from build123d import *

# Parameters (mm, degrees)
F0_R            = 60.325
F0_R_2          = 12.5
F1_DEPTH        = 10
F2_DEPTH        = 12.5
F3_DEPTH        = 12.5
F3_COPIES_COUNT = 26
F4_R            = 12.5
F5_DEPTH        = 22.501
F5_COPIES_COUNT = 5


# Not quite as in the source:
# - a pattern or mirror of a feature is missing from the dataset's text; its kind, count and spacing are read off the source's solid


with BuildPart() as f1:
    # F0 (on Front) → F1 (new body, symmetric)
    with BuildSketch(Plane.XZ):
        with BuildLine():
            ThreePointArc((-5.9714194874, 63.2186060373), (-42.7379507145, -46.9650675367), (63.5, 0))
            ThreePointArc((63.5, 0), (47.6226622583, 42.0039526644), (7.9304869469, 63.0028362598))
            ThreePointArc((7.9304869469, 63.0028362598), (0.9854569889, 63.4923528822), (-5.9714194874, 63.2186060373))
        make_face()
        Circle(F0_R, mode=Mode.SUBTRACT)
        Circle(F0_R)
        Circle(F0_R_2, mode=Mode.SUBTRACT)
    extrude(amount=F1_DEPTH, both=True)

    # F0 (on Front) → F2 (join, symmetric)
    with BuildSketch(Plane.XZ):
        with BuildLine():
            ThreePointArc((-5.9714194874, 63.2186060373), (-42.7379507145, -46.9650675367), (63.5, 0))
            ThreePointArc((63.5, 0), (47.6226622583, 42.0039526644), (7.9304869469, 63.0028362598))
            ThreePointArc((7.9304869469, 63.0028362598), (0.9854569889, 63.4923528822), (-5.9714194874, 63.2186060373))
        make_face()
        Circle(F0_R, mode=Mode.SUBTRACT)
    extrude(amount=F2_DEPTH, both=True)

    # F0 (on Front) → F3 (join, symmetric)
    with BuildSketch(Plane.XZ):
        with BuildLine():
            ThreePointArc((-5.9714194874, 63.2186060373), (0.9854569889, 63.4923528822), (7.9304869469, 63.0028362598))
            Line((7.9304869469, 63.0028362598), (2.54, 78.4059613943))
            Line((2.54, 78.4059613943), (0, 78.4059613943))
            Line((0, 78.4059613943), (-5.9714194874, 63.2186060373))
        make_face()
    f3 = extrude(amount=F3_DEPTH, both=True)

    # F3_copies: F3 ×26 about axis
    f3_copies_axis = Axis((0, 0, 0), (0, 1, 0))
    for i in range(1, F3_COPIES_COUNT):
        add(f3.rotate(f3_copies_axis, i * 360 / F3_COPIES_COUNT))

    # F4 (on face) → F5 (cut, through all)
    with BuildSketch(Plane.XZ.offset(10)):
        with Locations((-30, 0)):
            Circle(F4_R)
    f5 = extrude(amount=-F5_DEPTH, mode=Mode.SUBTRACT)

    # F5_copies: F5 ×5 about axis
    f5_copies_axis = Axis((0, 0, 0), (0, 1, 0))
    for i in range(1, F5_COPIES_COUNT):
        add(f5.rotate(f5_copies_axis, i * 360 / F5_COPIES_COUNT), mode=Mode.SUBTRACT)


solid = f1.part
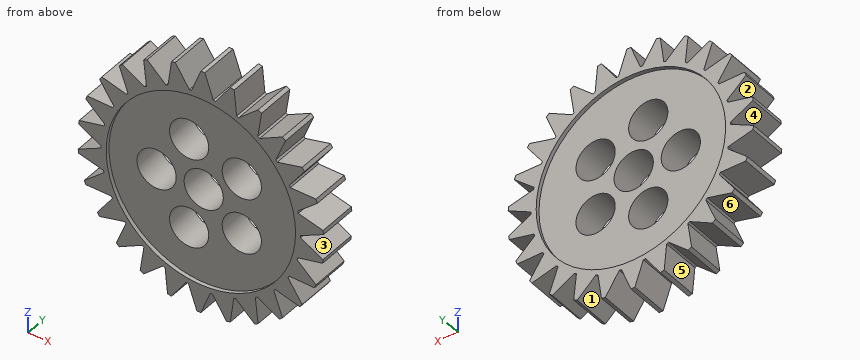
Can you work these out from the model? Positions are in its coordinate system, mm. Face numbers are marked on the shaded views. A direction names the side the tool comes from. Coordinates: 2 decimals unless noted, no trailing zeros. Write each loop counter-clockwise with the first axis right and the second up, starting at its lowest first coordinate (ties: lowest second). Pieces come first, ordered by that corner, then holes. Notation, with made-up numbers: (17, -7.5) -> (51, -7.5) arc R4 cw to (51, -3.5) -> close; hole circle Ø2 at (84.25, 53). An arc over 180 degrees is marked (long way). Write item = value, one per line.
(1) Imagine slicing it at B-B (y = 0). State how many separate pieces and enclosed holes the cut face has, and give its area (3 significant figures).
Verdict:
separate_pieces = 1
enclosed_holes = 6
area = 12,900 mm^2
(2) For pin 1 (8 mm diameter, centred on x = 56.5, y = -0.5, fed in from +Z); pin 2 (12 mm diameter, centred on x = 22.5, y = -5, fed in from -Z); pin 3 (1.5 mm diameter, centred on y = -8, z = 3.5, fed in from -X), each with a flat end and sliding along its axis, tell me the tip position at first contact or that it passes through.
Verdict:
pin_1 = 58.24
pin_2 = -76.69
pin_3 = -68.21
(3) If I drill on probe 1 along X at (y, z) = (0.75, 1); probe 2 along Z at (x, y) = (-58, -4.5); probe 3 along Z at (x, y) = (-57, 4.25), over which ranges is the centre line in solid material (lowest first)?
Verdict:
probe_1 = -63.49 to -42.46, -17.54 to -12.46, 12.46 to 66.1
probe_2 = -43.01 to -31.52, -27.99 to 29.81, 34.83 to 45.24
probe_3 = -42.78 to -30.15, -28 to 29.78, 33.35 to 44.96
(4) Imagine slicing it at A-A (x = -30). Please give me the cut outline in (y, z), and give its area (3 significant figures).
Verdict:
outline = (-12.5, -63.86) -> (12.5, -63.86) -> (12.5, -52.34) -> (10, -52.34) -> (10, -12.5) -> (-10, -12.5) -> (-10, -52.34) -> (-12.5, -52.34) -> close; (-12.5, 52.34) -> (-10, 52.34) -> (-10, 12.5) -> (10, 12.5) -> (10, 52.34) -> (12.5, 52.34) -> (12.5, 66.7) -> (-12.5, 66.7) -> close
area = 2,240 mm^2
(5) Imagine slicing it at C-C (x = 43.5). Please give me the cut outline in (y, z), and give its area (3 significant figures).
Verdict:
outline = (-12.5, -56.69) -> (12.5, -56.69) -> (12.5, -41.8) -> (10, -41.8) -> (10, 41.8) -> (12.5, 41.8) -> (12.5, 54.36) -> (-12.5, 54.36) -> (-12.5, 41.8) -> (-10, 41.8) -> (-10, -41.8) -> (-12.5, -41.8) -> close
area = 2,360 mm^2
(6) Thinking about a two-plate mould opening in X: for the marked faces 1, 2 and 3, which applies, +X half, -X half, draft (parallel to the pull), parting line (faces both ways), or undercut?
Verdict:
face_1 = undercut
face_2 = -X half
face_3 = +X half
(7) On a 3-axis mill with a long thin cutter (end or side, diameter ignored), from which of +Z, -Z, +X, -X, +Y, -Y can I reach the whole of each face in a straight line? I mean the marked faces 4, 5 and 6. Say none if no direction works.
Verdict:
face_4 = -X, +Y, -Y
face_5 = -Z, +Y, -Y
face_6 = +Y, -Y
